from build123d import *

# Parameters (mm, degrees)
SKETCH_1_R            = 2.84
EXTRUDE_261_DEPTH     = 3
SKETCH_2_R            = 1.5
EXTRUDE_345_DEPTH     = 4
CUT_EXTRUDE_529_DEPTH = 1.3
CHAMFER_591_SIZE      = 0.1


with BuildPart() as part:
    # 草图1 → Extrude 261 (new body)
    with BuildSketch(Plane(origin=(0, 0, 0), x_dir=(1, 0, 0), z_dir=(0, 1, 0))):
        with Locations(Location((0, 0, 0), (0, 0, 270))):
            Circle(SKETCH_1_R)
    extrude(amount=EXTRUDE_261_DEPTH)

    # 草图2 → Extrude 345 (add)
    with BuildSketch(Plane(origin=(0, 3, 0), x_dir=(1, 0, 0), z_dir=(0, 1, 0))):
        with Locations(Location((0, 0, 0), (0, 0, 270))):
            Circle(SKETCH_2_R)
    extrude(amount=EXTRUDE_345_DEPTH)

    # 草图3 → Cut-Extrude 529 (cut)
    with BuildSketch(Plane.XZ):
        Polygon((1.29, -0.744781847), (1.29, 0.744781847), (0, 1.489563695), (-1.29, 0.744781847), (-1.29, -0.744781847), (0, -1.489563695), align=None)
    extrude(amount=-CUT_EXTRUDE_529_DEPTH, mode=Mode.SUBTRACT)

    # Chamfer 591
    chamfer_591_edges = [part.edges().sort_by_distance(p)[0] for p in [
        (0, 0, -2.84),
        (0, 3, -2.84),
        (0, 7, -1.5),
    ]]
    chamfer(chamfer_591_edges, length=CHAMFER_591_SIZE)


solid = part.part
Geometry check sheet. Reference: the model listing, model coordinates, mm. A direction names the side the tool comes from. Give positions to 0.01 mm unless a question says otherwise; leave off trailing zeros. Order: outer loops, then holes, each group sorted by start corner. A loop starts at its lowest first (then second) coordinate and runs counter-clockwise, first axis right, second up.
1. Access from +Z, -Z, +X, -X, +Y, -Y to the whole of each face (thin tool, end or side, straight path). Record for faces 4 (the face through (-1.2, 3, 1.2)), 5 (the face through (1.29, 1, 0)), 6 (the face through (-1.2, 0, 1.2)).
Completed:
face 4: +Y
face 5: -Y
face 6: +Z, -Z, +X, -X, -Y
2. Depth check by flat-ended pin: pin 1 (1.3 mm diameter, centred on x = 0, z = -0.5, fed in from -Y); pin 2 (0.6 mm diameter, centred on y = 1, z = -0.5, fed in from +X); pin 3 (1.5 mm diameter, centred on y = 5.5, z = -0.5, fed in from +X). Enter the tip coordinate at first touch or a pass-through.
Completed:
pin 1: stops at y = 1.3
pin 2: stops at x = 2.83
pin 3: stops at x = 1.5
3. Draft check along Z on faces 1 (the face through (0.64, 0.64, -1.12)), 2 (the face through (0.45, 4.92, 1.43)), 3 (the face through (0, 7, 0)). Enter one of: pulls with the +Z half, pulls with the -Z half, needs draft (parallel to the pull), parting line crosses it, or undercut.
Completed:
face 1: undercut
face 2: parting line crosses it
face 3: needs draft
4. Scan lines: line 1 (X direction, y = 6.5, z = 0); line 2 (X direction, y = 1, z = -0.3); line 3 (Y direction, x = -2, z = 0.25). Record each from-to range of solid material in increasing order.
Completed:
line 1: x = -1.5 to 1.5
line 2: x = -2.82 to -1.29, 1.29 to 2.82
line 3: y = 0 to 3
5. Sectioned sample at B-B (y = 3.75). Record the boundary of the cut face in (x, z).
Completed:
outline: circle Ø3 at (0, 0)
6. Sectioned sample at A-A (z = 0). Record the boundary of the cut face in (x, y).
Completed:
outline: (-2.84, 0.1) - (-2.74, 0) - (-1.29, 0) - (-1.29, 1.3) - (1.29, 1.3) - (1.29, 0) - (2.74, 0) - (2.84, 0.1) - (2.84, 2.9) - (2.74, 3) - (1.5, 3) - (1.5, 6.9) - (1.4, 7) - (-1.4, 7) - (-1.5, 6.9) - (-1.5, 3) - (-2.74, 3) - (-2.84, 2.9) - close
